Geometry check sheet. Reference: the model listing, model coordinates, mm. A direction names the side the tool comes from. Round coordinates to 2 decimals unless told otherwise and drop trailing zeros. Write each loop counter-clockwise with the first axis right and the second up, starting at its lowest first coordinate (ties: lowest second). Pieces come first, ordered by that corner, then holes.
Item 1: Scan lines: probe 1 along X at (y, z) = (9.5, 18); probe 2 along X at (y, z) = (-13, 33); probe 3 along Z at (x, y) = (21.5, -5.5). Record each from-to range of solid material in increasing order.
Item 2: Cross-section at A-A (x = 19.5). Enter the section's corners in (y, z).
Item 3: Depth check by flat-ended pin: P1, Ø3, axis at x = 22.5, z = 29.5, coming from the +Y side; P2, Ø10, axis at x = 4.5, y = -2, coming from the +Z side; P3, Ø3, axis at x = 14.5, y = 12, coming from the -Z side; P4, Ø5, axis at x = 19.5, z = 5.5, coming from the +Y side. Enter the tip coordinate at first touch or a pass-through.
Item 4: Access from +Z, -Z, +X, -X, +Y, -Y to the whole of each face (thin tool, end or side, straight path). Record for faces 5 (the face through (-13, 2, 21.133)), 6 (the face through (22.13, 0.72, 48.84)), 7 (the face through (32.55, 13.4, 30.2)), 8 (the face through (13.35, 0.59, 9)).
Item 5: Draft check along X on faces 1 (the face through (14.288, -3, 42)), 2 (the face through (3.14, 9.04, 18.263)), 3 (the face through (2.3, 13.4, 0)), 4 (the face through (-15.554, 4.898, 10.418)). Enter one of: pulls with the +X half, pulls with the -X half, needs draft (parallel to the pull), parting line crosses it, or undercut.
Autodesk Inventor part; units mm, degrees
ref_plane "YZ Plane" through (0, 0, 0) normal (1, 0, 0) x (0, 1, 0)
ref_plane "XZ Plane" through (0, 0, 0) normal (0, 1, 0) x (-1, 0, 0)
ref_plane "XY Plane" through (0, 0, 0) normal (0, 0, 1) x (1, 0, 0)
sketch "Sketch1" plane through (0, 0, 0) normal (0, 1, 0) x (-1, 0, 0)
  line L0 (0, 0) -> (0, 18.2626)
  arc A0 (0, 18.2626) -> (-14.2875, 32.5501) centre (-14.2875, 18.2626) ccw
  line L1 (-14.2875, 32.5501) -> (-32.5501, 32.5501)
  line L2 (-14.2875, 32.5501) -> (0, 32.5501) construction
  line L3 (0, 32.5501) -> (0, 18.2626) construction
  dimension "d0" = 32.5501
  dimension "d1" = 32.5501
  dimension "d2" = 18.2626
sketch "Sketch2" plane through (0, 0, 0) normal (0, 0, 1) x (1, 0, 0)
  circle A0 centre (0, 0) radius 12.9794
  circle A1 centre (0, 0) radius 9.398
  dimension "d3" = 18.796
  dimension "d4" = 25.9588
sweep "Sweep1" add profiles "Sketch2" path "Sketch1"
sketch "Sketch3" plane through (0, 0, 0) normal (0, 0, -1) x (-1, 0, 0)
  circle A0 centre (0, 0) radius 16.3068
  circle A1 centre (0, 0) radius 12.9794
  circle A2 centre (0, 0) radius 11.1887
  dimension "d6" = 32.6136
  dimension "d9" = 22.3774
extrude "Extrusion1" add sketch "Sketch3" against normal blind 21.1328 contours A0 | A1
sketch "Sketch4" plane through (32.5501, 0, 32.5501) normal (1, 0, 0) x (0, 0, -1)
  circle A0 centre (0, 0) radius 9.398
  circle A1 centre (0, 0) radius 11.1887
  circle A2 centre (0, 0) radius 16.3068
  dimension "d10" = 32.6136
  dimension "d11" = 22.3774
extrude "Extrusion2" add sketch "Sketch4" against normal blind 21.1328 contours A2
sketch "Sketch5" plane through (0, 0, 0) normal (0, 0, -1) x (-1, 0, 0)
  circle A0 centre (0, 0) radius 9.398
  circle A1 centre (0, 0) radius 13.4366
  dimension "d14" = 26.8732
sketch "Sketch5 outline for Extrusion3" plane through (0, 0, 0) normal (0, 0, -1) x (-1, 0, 0)
  circle A0 centre (0, 0) radius 13.4366
extrude "Extrusion3" cut sketch "Sketch5 outline for Extrusion3" against normal blind 18.2626 draft -0.47812
sketch "Sketch6" plane through (32.5501, 0, 32.5501) normal (1, 0, 0) x (0, 0, -1)
  circle A0 centre (0, 0) radius 9.398
  circle A1 centre (0, 0) radius 13.4366
  dimension "d17" = 26.8732
sketch "Sketch6 outline for Extrusion4" plane through (32.5501, 0, 32.5501) normal (1, 0, 0) x (0, 0, -1)
  circle A0 centre (0, 0) radius 13.4366
extrude "Extrusion4" cut sketch "Sketch6 outline for Extrusion4" against normal blind 18.2626 draft -0.47812
equation "\"d0\" = G + C1"
equation "\"d1\" = G + C1"
equation "\"d2\" = C1"
equation "\"d3\" = D"
equation "\"d4\" = D + 2 * F1"
equation "\"d6\" = A + 2 * E1"
equation "\"d9\" = D + F1"
equation "\"d7\" = C1 + E1"
equation "\"d10\" = A + 2 * E1"
equation "\"d11\" = D + F1"
equation "\"d12\" = C1 + E1"
equation "\"d14\" = A"
equation "\"d15\" = C1"
equation "\"d17\" = A"
equation "\"d18\" = C1"
equation "\"A\" = 26.8732"
equation "\"C1\" = 18.2626"
equation "\"F1\" = 3.5814"
equation "\"D\" = 18.796"
equation "\"G\" = 14.2875"
equation "\"E1\" = 2.8702"
equation "\"B\" = 26.5684"
equation "\"Size_Designation\" = 0.75"
properties part number "ASTM D 2466 90 Deg Elbow Socket-Type - Schedule 40 3/4" material "PVC-Piping"
Resolved:
1. probe 1: x = -13.25 to -9.29, 9.29 to 13.25
1. probe 2: x = 11.42 to 14.29
1. probe 3: z = 17.2 to 20.39, 44.71 to 47.9
2. outline: circle Ø32.61 at (0, 32.55); hole circle Ø26.66 at (0, 32.55)
3. P1: stops at y = 16.23
3. P2: stops at z = 45.06
3. P3: stops at z = 20.07
3. P4: passes through
4. face 5: none
4. face 6: +X
4. face 7: +Z, -Z, +X, +Y, -Y
4. face 8: -Z
5. face 1: pulls with the +X half
5. face 2: undercut
5. face 3: needs draft
5. face 4: parting line crosses it
